Work out the finished part from the listing and answer in its coordinate system (mm). Face numbers are marked on the shaded views. A direction names the side the tool comes from. Coordinates: 2 decimals unless noted, no trailing zeros. Order: outer loops, then holes, each group sorted by start corner. A loop starts at its lowest first (then second) coordinate and runs counter-clockwise, first axis right, second up. Notation, with made-up numbers: M -3.75,29.5 L 42.25,29.5 A27 cw 42.25,57.5 Z; hole C 23,-33 d2. An arc over 180 degrees is marked long. Use a Markdown table: item, result.
from build123d import *

# Parameters (mm, degrees)
SZKIC1_W                    = 69.7
SZKIC1_H                    = 80
DODANIE_WYCI_GNI_CIE1_DEPTH = 15
SZKIC3_R                    = 3
WYTNIJ_WYCI_GNI_CIE1_DEPTH  = 15
SZKIC4_R                    = 5
WYTNIJ_WYCI_GNI_CIE2_DEPTH  = 7
SZKIC5_R                    = 3
WYTNIJ_WYCI_GNI_CIE3_DEPTH  = 15


with BuildPart() as part:
    # Szkic1 → Dodanie-wyciągnięcie1 (new body)
    with BuildSketch(Plane.XY):
        Rectangle(SZKIC1_W, SZKIC1_H)
    extrude(amount=DODANIE_WYCI_GNI_CIE1_DEPTH)

    # Szkic3 → Wytnij-wyciągnięcie1 (cut)
    with BuildSketch(Plane(origin=(0, 0, 0), x_dir=(1, 0, 0), z_dir=(0, 0, -1))):
        with Locations((12.85, 33)):
            Circle(SZKIC3_R)
        with Locations((-3.15, 33)):
            Circle(SZKIC3_R)
        with Locations((-3.15, -33)):
            Circle(SZKIC3_R)
        with Locations((12.85, -33)):
            Circle(SZKIC3_R)
    extrude(amount=-WYTNIJ_WYCI_GNI_CIE1_DEPTH, mode=Mode.SUBTRACT)

    # Szkic4 → Wytnij-wyciągnięcie2 (cut)
    with BuildSketch(Plane(origin=(0, 0, 0), x_dir=(-1, 0, 0), z_dir=(0, 0, 1))):
        with Locations((3.15, 33)):
            Circle(SZKIC4_R)
        with Locations((-12.85, 33)):
            Circle(SZKIC4_R)
        with Locations((-12.85, -33)):
            Circle(SZKIC4_R)
        with Locations((3.15, -33)):
            Circle(SZKIC4_R)
    extrude(amount=WYTNIJ_WYCI_GNI_CIE2_DEPTH, mode=Mode.SUBTRACT)

    # Szkic5 → Wytnij-wyciągnięcie3 (cut)
    with BuildSketch(Plane.XY.offset(15)):
        with Locations((-27.85, 33)):
            Circle(SZKIC5_R)
        with Locations((27.85, 33)):
            Circle(SZKIC5_R)
        with Locations((27.85, -33)):
            Circle(SZKIC5_R)
        with Locations((-27.85, -33)):
            Circle(SZKIC5_R)
    extrude(amount=-WYTNIJ_WYCI_GNI_CIE3_DEPTH, mode=Mode.SUBTRACT)


solid = part.part
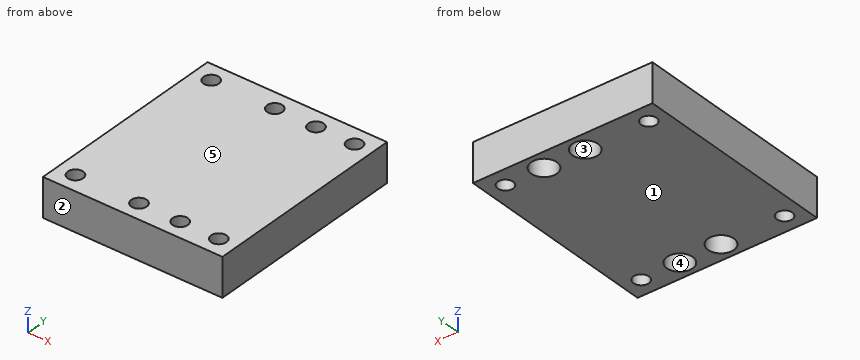
1. Section A-A on x = -3.15 is taken. Determine the outline of the cut face in (y, z), then the cut area to 3 significant figures.
Answers below:
| item | result |
|---|---|
| outline | M -40,0 L -38,0 L -38,7 L -36,7 L -36,15 L -40,15 Z; M -30,7 L -28,7 L -28,0 L 28,0 L 28,7 L 30,7 L 30,15 L -30,15 Z; M 36,7 L 38,7 L 38,0 L 40,0 L 40,15 L 36,15 Z |
| area | 964 mm² |
2. Find the intervals of material crossed by probe 1 along Y at (x, z) = (-3.15, 10.75); probe 2 along Y at (x, z) = (12.85, 1.5), in increasing order.
Answers below:
| item | result |
|---|---|
| probe 1 | -40 to -36, -30 to 30, 36 to 40 |
| probe 2 | -40 to -38, -28 to 28, 38 to 40 |
3. Section B-B on z = 10.5 is taken. Give the number of separate pieces and of enclosed holes in the cut face, then the cut area to 3 significant figures.
Answers below:
| item | result |
|---|---|
| separate pieces | 1 |
| enclosed holes | 8 |
| area | 5,350 mm² |
4. A flat-ended cylindrical pin translates along its axis: P1, Ø8, axis at x = -3.15, y = 33, coming from the -Z side. Find the tip coordinate at first contact, or state that the pin passes through.
Answers below:
| item | result |
|---|---|
| P1 | z = 7 |
5. Section C-C on y = 33 is taken. Determine the outline of the cut face in (x, z), then the cut area to 4 significant figures.
Answers below:
| item | result |
|---|---|
| outline | M -34.85,0 L -30.85,0 L -30.85,15 L -34.85,15 Z; M -24.85,0 L -8.15,0 L -8.15,7 L -6.15,7 L -6.15,15 L -24.85,15 Z; M -0.15,7 L 1.85,7 L 1.85,0 L 7.85,0 L 7.85,7 L 9.85,7 L 9.85,15 L -0.15,15 Z; M 15.85,7 L 17.85,7 L 17.85,0 L 24.85,0 L 24.85,15 L 15.85,15 Z; M 30.85,0 L 34.85,0 L 34.85,15 L 30.85,15 Z |
| area | 629.5 mm² |
6. For the marked faces 4 and 5, determine the directions among +Z, -Z, +X, -X, +Y, -Y from which every point of the face is accessible in a straight line to the end or side of a thin tool.
Answers below:
| item | result |
|---|---|
| face 4 | -Z |
| face 5 | +Z, +X, -X, +Y, -Y |
7. For a pull along Y with two mould halves and no side action, classify the marked faces 1, 2 and 3 as +Y half, -Y half, draft (parallel to the pull), parting line (faces both ways), or undercut.
Answers below:
| item | result |
|---|---|
| face 1 | draft |
| face 2 | -Y half |
| face 3 | undercut |
